Study the drawing (mm; zero at the part's minimum x, y, z) and answer. A direction names the side the tool comes from. Give positions to 0.01 mm unless a question says otherwise; leave off trailing zeros. Order: outer loops, then holes, each group sorted by start corner. A loop starts at its lowest first (then second) coordinate and runs counter-clockwise, first axis right, second up. Notation, with made-up numbers: (17, 3) - (22, 3) arc R30 cw to (22, 39) - close; hole circle Ø11 at (36, 17.25). An arc over 180 degrees is marked (long way). Write each question's results on one line, items separated by ' | '. Start each with the question number.
Q1. A flat-ended cylindrical pin translates along its axis: P1, Ø3, axis at x = 4, z = 11, coming from the -Y side. Find the tip coordinate at first contact, or state that the pin passes through.
Q2. A tool of negligible diameter and unlimited length cuts with its end or side. For the marked faces 4 and 5, from which of +Z, -Z, +X, -X, +Y, -Y can it reach the whole face along a straight path? Write none if from no direction.
Q3. For a pull along X with two mould halves and no side action, classify the marked faces 1, 2 and 3 as +X half, -X half, draft (parallel to the pull), parting line (faces both ways), or undercut.
Q4. Find section B-B on x = 14.5. Give the vertices of the cut face in (y, z), and give its area (3 significant figures).
Q5. Find section C-C on y = 5. Give the vertices of the cut face in (x, z), and give its area (3 significant figures).
Q6. Find section A-A on z = 12.1. Give the vertices of the cut face in (x, y).
Q7. Find the intervals of material crossed by line 1 along Z through (x, y) = (7.25, 24); line 2 along Y through (x, z) = (9.5, 17.25), in increasing order. Write a range as from..to.
Q8. Find section D-D on y = 27. Give the vertices of the cut face in (x, z), and give its area (3 significant figures).
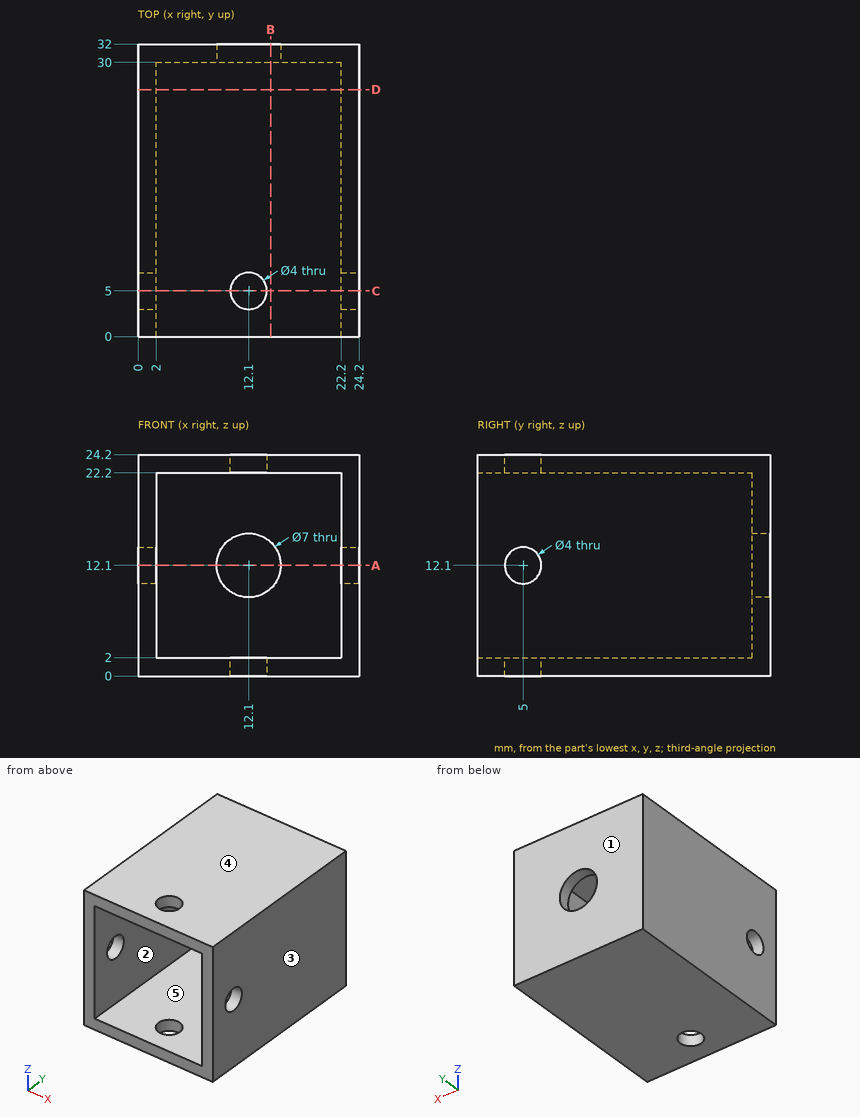
Working result:
1) P1: y = 30
2) face 4: +Z, +X, -X, +Y, -Y | face 5: -Y
3) face 1: draft | face 2: undercut | face 3: +X half
4) outline: (0, 0) - (32, 0) - (32, 9.55) - (30, 9.55) - (30, 2) - (0, 2) - close; (0, 22.2) - (30, 22.2) - (30, 14.65) - (32, 14.65) - (32, 24.2) - (0, 24.2) - close | area: 158 mm²
5) outline: (0, 0) - (10.1, 0) - (10.1, 2) - (2, 2) - (2, 10.1) - (0, 10.1) - close; (0, 14.1) - (2, 14.1) - (2, 22.2) - (10.1, 22.2) - (10.1, 24.2) - (0, 24.2) - close; (14.1, 0) - (24.2, 0) - (24.2, 10.1) - (22.2, 10.1) - (22.2, 2) - (14.1, 2) - close; (14.1, 22.2) - (22.2, 22.2) - (22.2, 14.1) - (24.2, 14.1) - (24.2, 24.2) - (14.1, 24.2) - close | area: 146 mm²
6) outline: (0, 0) - (2, 0) - (2, 3) - (0, 3) - close; (0, 7) - (2, 7) - (2, 30) - (8.6, 30) - (8.6, 32) - (0, 32) - close; (15.6, 30) - (22.2, 30) - (22.2, 7) - (24.2, 7) - (24.2, 32) - (15.6, 32) - close; (22.2, 0) - (24.2, 0) - (24.2, 3) - (22.2, 3) - close
7) line 1: 0..2, 22.2..24.2 | line 2: 30..32
8) outline: (0, 0) - (24.2, 0) - (24.2, 24.2) - (0, 24.2) - close; hole (2, 2) - (22.2, 2) - (22.2, 22.2) - (2, 22.2) - close | area: 178 mm²
